Geometry check sheet. Reference: the model listing, model coordinates, mm. A direction names the side the tool comes from. Coordinates: 2 decimals unless noted, no trailing zeros. Write each loop counter-clockwise with the first axis right and the second up, starting at its lowest first coordinate (ties: lowest second). Pieces come first, ordered by that corner, then holes. Notation, with made-up numbers: M 56.5,12.5 L 107.5,12.5 A21 ccw 107.5,16.5 Z; hole C 67.25,19 d4. An arc over 180 degrees is marked long. Answer as a JSON object with one key per item and string values. Group by question number.
Autodesk Inventor part; units mm, degrees
ref_plane "YZ Plane" through (0, 0, 0) normal (1, 0, 0) x (0, 1, 0)
ref_plane "XZ Plane" through (0, 0, 0) normal (0, 1, 0) x (-1, 0, 0)
ref_plane "XY Plane" through (0, 0, 0) normal (0, 0, 1) x (1, 0, 0)
sketch "Skizze1" plane through (0, 0, 0) normal (0, 0, 1) x (1, 0, 0)
  line L0 (-20, -20) -> (20, -20)
  line L1 (20, -20) -> (20, 20)
  line L2 (20, 20) -> (-20, 20)
  line L3 (-20, 20) -> (-20, -20)
  line L4 (-20, -20) -> (20, 20) construction
  line L5 (20, -20) -> (-20, 20) construction
  point P0 (0, 0)
  dimension "d0" = 40
  dimension "d1" = 40
extrude "Extrusion1" add sketch "Skizze1" along normal blind 5
sketch "Skizze2" plane through (-20, -20, 0) normal (-1, 0, 0) x (0, 0, 1)
  line L0 (5, 40) -> (5, 0)
  line L1 (0, 0) -> (40, 0)
  line L2 (40, 0) -> (40, 40)
  line L3 (40, 40) -> (0, 40)
  line L4 (0, 40) -> (0, 0)
  point P0 (0, 20)
  dimension "d4" = 40
  dimension "d5" = 40
extrude "Extrusion2" add sketch "Skizze2" against normal blind 5 contours L3 L2 L1 L0
sketch "Skizze3" plane through (-20, 20, 0) normal (0, 1, 0) x (1, 0, 0)
  line L0 (40, 0) -> (0, 0)
  line L1 (0, 0) -> (0, -40)
  line L2 (5, -5) -> (5, -40)
  line L3 (40, -5) -> (5, -5)
  line L4 (0, 0) -> (40, 0)
  line L5 (40, 0) -> (40, -40)
  line L6 (40, -40) -> (0, -40)
  line L7 (0, -40) -> (0, 0)
  point P0 (20, 0)
  point P1 (5, -40)
  point P2 (0, -5)
  dimension "d8" = 40
  dimension "d9" = 40
extrude "Extrusion3" add sketch "Skizze3" against normal blind 5 contours L5 L6 L2 L3
sketch "Skizze4" plane through (-15, -20, 0) normal (1, 0, 0) x (0, 0, -1)
  line L0 (-5, 35) -> (-40, 35)
  line L1 (-40, 40) -> (-40, 0)
  line L2 (-40, 0) -> (-5, 0)
  line L3 (-5, 40) -> (-5, 0)
  point P0 (0, 20)
  point P1 (-33, 28)
  point P2 (-12, 7)
  dimension "d12" = 7
  dimension "d13" = 7
  dimension "d14" = 7
  dimension "d15" = 7
hole "Bohrung1" at (-15, 8, 33) at (-15, -13, 12) direction (-1, 0, 0) diameter 6.1 end through all
sketch "Skizze5" plane through (-20, 15, 0) normal (0, -1, 0) x (1, 0, 0)
  line L0 (40, 5) -> (40, 40)
  line L1 (40, 40) -> (5, 40)
  line L2 (5, 5) -> (5, 40)
  line L3 (40, 5) -> (5, 5)
  point P0 (20, 0)
  point P1 (12, 33)
  point P2 (33, 12)
  dimension "d23" = 7
  dimension "d24" = 7
  dimension "d25" = 7
  dimension "d26" = 7
hole "Bohrung2" at (-8, 15, 33) at (13, 15, 12) direction (0, 1, 0) diameter 6.1 end through all
sketch "Skizze6" plane through (0, 0, 5) normal (0, 0, 1) x (1, 0, 0)
  line L0 (20, 15) -> (-15, 15)
  line L1 (-15, 15) -> (-15, -20)
  line L2 (-15, -20) -> (20, -20)
  line L3 (20, -20) -> (20, 15)
  point P0 (0, 0)
  point P1 (-8, -13)
  point P2 (13, 8)
  dimension "d34" = 7
  dimension "d35" = 7
  dimension "d36" = 7
  dimension "d37" = 7
hole "Bohrung3" at (-8, -13, 5) at (13, 8, 5) direction (0, 0, -1) diameter 6.1 end through all
equation "\"d5\" = d4"
equation "\"d8\" = d9"
properties part number "Ecken_Box"
1) Material ranges on probe 1 along Z at (x, y) = (13, 17.4); probe 2 along Y at (x, z) = (-8, 1.45); probe 3 along X at (y, z) = (18.3, 12), recorded low to high. Write a range as [from, to].
2) Section check C-C (z = 21.5). Record the cut outline in (x, y), then the cut area to 3 significant figures.
3) Draft check along Z on faces 3 (the cylindrical face through (10.94, 10.25, 2.46)), 4 (the cylindrical face through (-17.535, 9.168, 30.183)), 5 (the flat face through (0, 0, 0)). Enter one of: +Z half, -Z half, draft (parallel to the pull), parting line (faces both ways), or undercut.
4) Go/stop test with flat-tipped pins: pin 1 Ø7 at (x, y) = (-8, -13) entering from +Z; pin 2 Ø1 at (x, y) = (-11.5, 1) entering from -Z; pin 3 Ø10.5 at (y, z) = (-1, 25) entering from +X; pin 4 Ø7 at (x, z) = (-8, 33) entering from -Y. Record where each tip stops, or that it passes through.
5) Set-up check for faces 1 (the flat face through (20, 9, 4)), 2 (the flat face through (2, -2, 5)): record each of +Z, -Z, +X, -X, +Y, -Y from which the full face is reachable in a straight line by a thin tool's end or side.
6) Section check B-B (y = -13). Record the cut outline in (x, z), then the cut area to 3 significant figures.
7) Section check A-A (z = 33). Record the cut outline in (x, y), then the cut area to 3 significant figures.
8) Section check D-D (x = 9). Record the cut outline in (y, z).
Entries:
{
 "1": {"probe 1": "[0, 8.95], [15.05, 40]", "probe 2": "[-20, -16.05], [-9.95, 20]", "probe 3": "[-20, 9.95], [16.05, 20]"},
 "2": {"outline": "M -20,-20 L -15,-20 L -15,15 L 20,15 L 20,20 L -20,20 Z", "area": "375 mm^2"},
 "3": {"face 3": "draft", "face 4": "undercut", "face 5": "-Z half"},
 "4": {"pin 1": "z = 5", "pin 2": "z = 0", "pin 3": "x = -15", "pin 4": "y = 15"},
 "5": {"face 1": "+Z, -Z, +X, +Y, -Y", "face 2": "+Z, +X, -Y"},
 "6": {"outline": "M -20,0 L -11.05,0 L -11.05,5 L -15,5 L -15,8.95 L -20,8.95 Z; M -20,15.05 L -15,15.05 L -15,40 L -20,40 Z; M -4.95,0 L 20,0 L 20,5 L -4.95,5 Z", "area": "314 mm^2"},
 "7": {"outline": "M -20,-20 L -15,-20 L -15,4.95 L -20,4.95 Z; M -20,11.05 L -15,11.05 L -15,15 L -11.05,15 L -11.05,20 L -20,20 Z; M -4.95,15 L 20,15 L 20,20 L -4.95,20 Z", "area": "314 mm^2"},
 "8": {"outline": "M -20,0 L 20,0 L 20,40 L 15,40 L 15,5 L -20,5 Z"}
}
